```python
from build123d import *

# Parameters (mm, degrees)
SKETCH1_R           = 63.5
SKETCH1_R_2         = 50.8
BOSS_EXTRUDE1_DEPTH = 114.3
SKETCH2_R           = 63.5
BOSS_EXTRUDE2_DEPTH = 6.35
CHAMFER1_SIZE       = 5.08
CHAMFER1_SIZE2      = 28.810111644
SKETCH3_R           = 15.875
CUT_EXTRUDE1_DEPTH  = 121.65
SKETCH4_R           = 10.795
BOSS_EXTRUDE3_DEPTH = 19.05
FILLET1_R           = 2.54


with BuildPart() as part:
    # Sketch1 → Boss-Extrude1 (new body)
    with BuildSketch(Plane(origin=(0, 0, 0), x_dir=(1, 0, 0), z_dir=(0, 1, 0))):
        Circle(SKETCH1_R)
        Circle(SKETCH1_R_2, mode=Mode.SUBTRACT)
    extrude(amount=BOSS_EXTRUDE1_DEPTH)

    # Sketch2 → Boss-Extrude2 (add)
    with BuildSketch(Plane(origin=(0, 114.3, 0), x_dir=(1, 0, 0), z_dir=(0, 1, 0))):
        Circle(SKETCH2_R)
    extrude(amount=BOSS_EXTRUDE2_DEPTH)

    # Chamfer1
    chamfer1_edges = [part.edges().sort_by_distance(p)[0] for p in [
        (-63.5, 120.65, 0),
    ]]
    chamfer1_side = [part.faces().sort_by_distance(p)[0] for p in [
        (-63.5, 60.325, 0),
    ]]
    chamfer(chamfer1_edges, length=CHAMFER1_SIZE, length2=CHAMFER1_SIZE2, reference=chamfer1_side[0])

    # Sketch3 → Cut-Extrude1 (cut, through all)
    with BuildSketch(Plane(origin=(0, 120.65, 0), x_dir=(1, 0, 0), z_dir=(0, 1, 0))):
        with Locations((0, 31.75)):
            Circle(SKETCH3_R)
        with Locations((30.196044392, 9.811289571)):
            Circle(SKETCH3_R)
        with Locations((18.66218176, -25.686289571)):
            Circle(SKETCH3_R)
        with Locations((-18.66218176, -25.686289571)):
            Circle(SKETCH3_R)
        with Locations((-30.196044392, 9.811289571)):
            Circle(SKETCH3_R)
    extrude(amount=-CUT_EXTRUDE1_DEPTH, mode=Mode.SUBTRACT)

    # Sketch4 → Boss-Extrude3 (add)
    with BuildSketch(Plane(origin=(0, 120.65, 0), x_dir=(1, 0, 0), z_dir=(0, 1, 0))):
        Circle(SKETCH4_R)
    extrude(amount=BOSS_EXTRUDE3_DEPTH)

    # Fillet1
    fillet1_edges = [part.edges().sort_by_distance(p)[0] for p in [
        (-10.795, 139.7, 0),
    ]]
    fillet(fillet1_edges, radius=FILLET1_R)


solid = part.part
```
Work out the finished part from the listing and answer in its coordinate system (mm). A direction names the side the tool comes from. Coordinates: 2 decimals unless noted, no trailing zeros. Write each loop counter-clockwise with the first axis right and the second up, starting at its lowest first coordinate (ties: lowest second). Pieces come first, ordered by that corner, then holes.
Q1. Each of these flat-tipped pins is pushed along its axis until it touches: pin 1 Ø5 at (x, z) = (15.5, 45) entering from +Y; pin 2 Ø2 at (x, y) = (19, 20) entering from -Z; pin 3 Ø3 at (x, y) = (-24, 58.5) entering from -Z. Where does it stop, or does it pass through?
Q2. Determine the mould class of faces 4 (the face through (-10.13, 117.52, 12.3)), 5 (the face through (-13.77, 56.98, 61.99)), 6 (the face through (-8, 120.65, -8)) for opening direction Z: released by +Z, released by -Z, zero draft, split by the parting line, or undercut.
Q3. A cutting plane is placed at A-A, the plane x = 0. Give the vertices of the cut face in (y, z) (3 decimals).
Q4. Find the intervals of material crossed by line 1 (X direction, y = 23.5, z = 2); line 2 (X direction, y = 109, z = -45); line 3 (Z direction, x = -11, y = 79.5), in increasing order.
Q5. A cutting plane is placed at D-D, the plane x = -18.5. State how many separate pieces and enclosed holes the cut face has, then the cut area to 3 significant figures.
Q6. A cutting plane is placed at C-C, the plane y = 19. Give the vertices of the cut face in (x, z), then the cut area to 3 significant figures.
Q7. A cutting plane is placed at B-B, the plane z = 0. Give the vertices of the cut face in (x, y) (3 decimals), then the cut area to 3 significant figures.
Q8. Which of the six approach directions +Z, -Z, +X, -X, +Y, -Y give full straight-line access (tool end or side, diameter ignored) to faces 1 (the face through (-1, 114.3, 11)), 2 (the face through (-7.956, 128.789, -7.296)), 3 (the face through (6.96, 117.52, 14.96))?
Findings below:
1. pin 1: stops at y = 118.82
1. pin 2: stops at z = -60.9
1. pin 3: stops at z = -59.38
2. face 4: undercut
2. face 5: split by the parting line
2. face 6: zero draft
3. outline: (0, -63.5) - (115.57, -63.5) - (118.369, -47.625) - (114.3, -47.625) - (114.3, -50.8) - (0, -50.8) - close; (0, 50.8) - (114.3, 50.8) - (114.3, -15.875) - (120.65, -15.875) - (120.65, -10.795) - (137.16, -10.795) arc R2.54 ccw to (139.7, -8.255) - (139.7, 8.255) arc R2.54 ccw to (137.16, 10.795) - (120.65, 10.795) - (120.65, 34.69) - (115.57, 63.5) - (0, 63.5) - close
4. line 1: x = -63.47 to -50.76, 50.76 to 63.47
4. line 2: x = -44.8 to -23.57, 23.57 to 44.8
4. line 3: z = -62.54 to -49.59, 49.59 to 62.54
5. separate pieces: 3
5. enclosed holes: 0
5. area: 3,360 mm2
6. outline: circle Ø127 at (0, 0); hole circle Ø101.6 at (0, 0)
6. area: 4,560 mm2
7. outline: (-63.5, 0) - (-50.8, 0) - (-50.8, 114.3) - (-42.676, 114.3) - (-42.676, 119.242) - (-63.5, 115.57) - close; (-17.716, 114.3) - (17.716, 114.3) - (17.716, 120.65) - (10.795, 120.65) - (10.795, 137.16) arc R2.54 ccw to (8.255, 139.7) - (-8.255, 139.7) arc R2.54 ccw to (-10.795, 137.16) - (-10.795, 120.65) - (-17.716, 120.65) - close; (42.676, 114.3) - (50.8, 114.3) - (50.8, 0) - (63.5, 0) - (63.5, 115.57) - (42.676, 119.242) - close
7. area: 3,670 mm2
8. face 1: -Y
8. face 2: +Y
8. face 3: +Y, -Y
